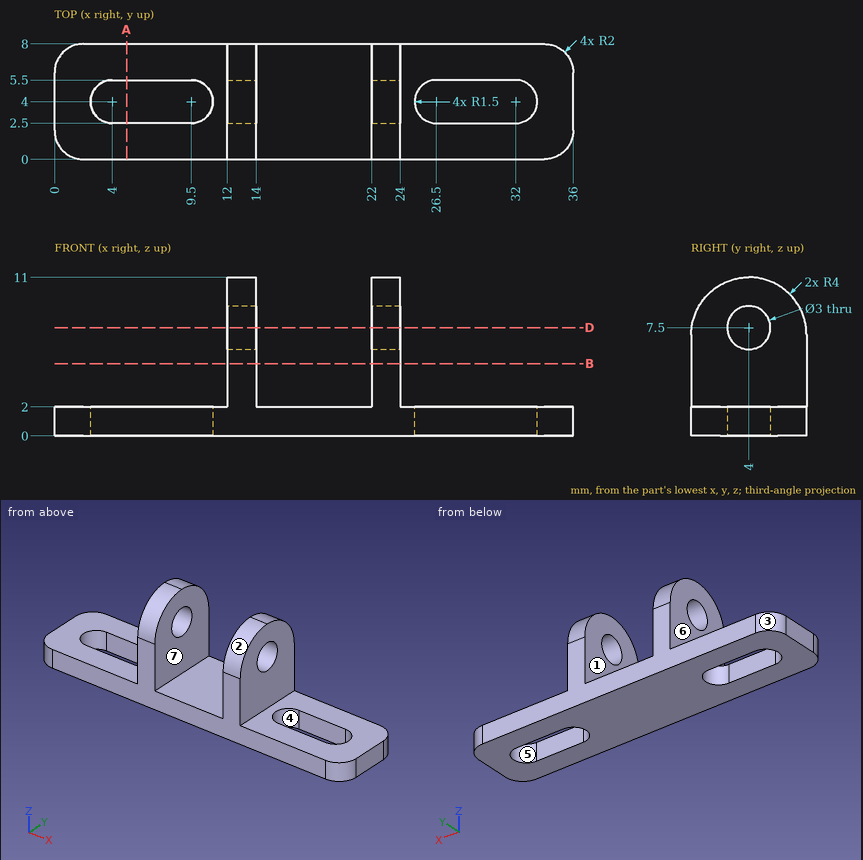
The drawing under review shows one solid part. Ordinate dimensions are in mm from its lowest x, y, z. A direction names the side the tool comes from. Round coordinates to 2 decimals unless told otherwise and drop trailing zeros. Write each loop counter-clockwise with the first axis right and the second up, starting at its lowest first coordinate (ties: lowest second). Pieces come first, ordered by that corner, then holes. Notation, with made-up numbers: (6, 56.5) -> (61, 56.5) arc R23 cw to (61, 79.5) -> close; hole circle Ø4 at (66, 33). An arc over 180 degrees is marked (long way). Put each result on its own line as item: value.
Q1. Consider section D-D on z = 7.5. State the section outline as (x, y) points.
Determined:
outline: (12, 0.03) -> (14, 0.03) -> (14, 2.5) -> (12, 2.5) -> close; (12, 5.5) -> (14, 5.5) -> (14, 7.97) -> (12, 7.97) -> close; (22, 0.03) -> (24, 0.03) -> (24, 2.5) -> (22, 2.5) -> close; (22, 5.5) -> (24, 5.5) -> (24, 7.97) -> (22, 7.97) -> close
Q2. Clearance check with flat-ended pins moving along their axes: pin 1 Ø2.5 at (x, y) = (19.5, 2.5) entering from +Z; pin 2 Ø2.5 at (y, z) = (2.5, 5) entering from +X; pin 3 Ø2.5 at (y, z) = (4, 7.5) entering from -X. State where each tip first meets the part, or that it passes through.
Determined:
pin 1: stops at z = 2
pin 2: stops at x = 24
pin 3: passes through
Q3. Consider section B-B on z = 5. State the section outline as (x, y) points.
Determined:
outline: (12, 0) -> (14, 0) -> (14, 8) -> (12, 8) -> close; (22, 0) -> (24, 0) -> (24, 8) -> (22, 8) -> close
Q4. Machinability: for the marked faces 5, 6 and 7, which of the approach directions +Z, -Z, +X, -X, +Y, -Y give a long, thin tool a straight path to every point of the face, cutting with its end or side? Answer none if there is none.
Determined:
face 5: +Z, -Z
face 6: +Z, -X, +Y, -Y
face 7: +Z, +Y, -Y
Q5. Consider section A-A on x = 5. State the section outline as (y, z) points.
Determined:
outline: (0, 0) -> (2.5, 0) -> (2.5, 2) -> (0, 2) -> close; (5.5, 0) -> (8, 0) -> (8, 2) -> (5.5, 2) -> close
Q6. To check wall thickness, follow L1, parallel to X at y = 5.25, z = 6; L2, parallel to Y at x = 5, z = 1.5; L3, parallel to Z at x = 23.45, y = 4. State the ranges of each line that lie inside material, in increasing order. Write a range as [from, to].
Determined:
L1: x = [12, 14], [22, 24]
L2: y = [0, 2.5], [5.5, 8]
L3: z = [0, 6], [9, 11]
Q7. The part is to be moulded in two halves that separate along Y. For the marked faces 1, 2, 3 and 4, say which applies: released by +Y, released by -Y, zero draft, split by the parting line, or undercut.
Determined:
face 1: zero draft
face 2: released by -Y
face 3: released by +Y
face 4: undercut
